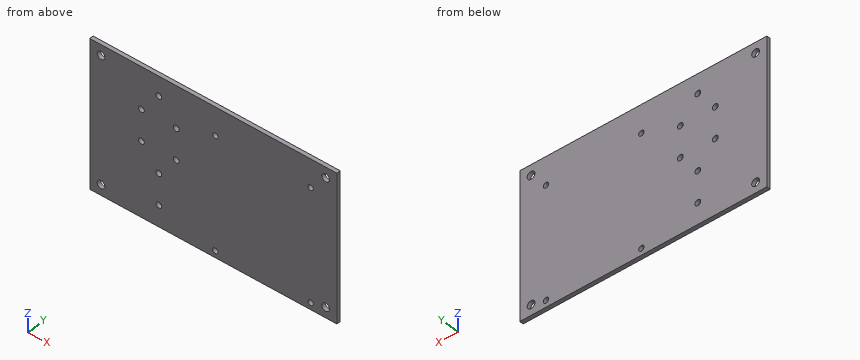
Autodesk Inventor part; units mm, degrees
ref_plane "YZ Plane" through (0, 0, 0) normal (1, 0, 0) x (0, 1, 0)
ref_plane "XZ Plane" through (0, 0, 0) normal (0, 1, 0) x (-1, 0, 0)
ref_plane "XY Plane" through (0, 0, 0) normal (0, 0, 1) x (1, 0, 0)
sketch "Sketch1" plane through (0, 0, 0) normal (0, 1, 0) x (-1, 0, 0)
  line L0 (0, 0) -> (-127, 0)
  line L1 (-127, 0) -> (-127, 76)
  line L2 (-127, 76) -> (0, 76)
  line L3 (0, 76) -> (0, 0)
  dimension "d0" = 76
  dimension "d1" = 127
extrude "Extrusion1" add sketch "Sketch1" along normal blind 2
sketch "Sketch2" plane through (0, 0, 0) normal (0, -1, 0) x (1, 0, 0)
  line L0 (0, 0) -> (127, 0)
  line L1 (127, 0) -> (127, 76)
  line L2 (127, 76) -> (0, 76)
  line L3 (0, 76) -> (0, 0)
  line L4 (0, 5.4) -> (127, 5.4) construction
  line L5 (0, 38) -> (127, 38) construction
  line L6 (63.5, 76) -> (63.5, 0) construction
  line L7 (121.2, 76) -> (121.2, 0) construction
  line L8 (0, 70.6) -> (127, 70.6) construction
  line L9 (5.8, 76) -> (5.8, 0) construction
  circle A0 centre (121.2, 70.6) radius 2
  circle A1 centre (121.2, 5.4) radius 2
  circle A2 centre (5.8, 70.6) radius 2
  circle A3 centre (5.8, 5.4) radius 2
  dimension "d5" = 32.6
  dimension "d6" = 57.7
  dimension "d7" = 4
extrude "Extrusion2" cut sketch "Sketch2" against normal through all contours A0 | A1 | A2 | A3
sketch "Sketch3" plane through (0, 0, 0) normal (0, -1, 0) x (1, 0, 0)
  line L0 (0, 0) -> (127, 0)
  line L1 (0, 76) -> (0, 0)
  line L2 (10, 93) -> (61, 93)
  line L3 (61, 93) -> (61, 0)
  line L4 (61, 0) -> (10, 0)
  line L5 (10, 0) -> (10, 93)
  line L6 (61, 0) -> (117, 0)
  line L7 (117, 0) -> (117, 85)
  line L8 (117, 85) -> (61, 85)
  line L9 (61, 85) -> (61, 0)
  line L10 (35.5, 93) -> (35.5, 0) construction
  circle A0 centre (35.5, 27) radius 1.5
  circle A1 centre (35.5, 82) radius 1.5
  line L11 (89, 85) -> (89, 0) construction
  line L12 (117, 42.5) -> (61, 42.5) construction
  circle A2 centre (113.5, 3.5) radius 1.375
  circle A3 centre (113.5, 61.5) radius 1.375
  circle A4 centre (64.5, 3.5) radius 1.375
  circle A5 centre (64.5, 61.5) radius 1.375
  line L13 (35.5, 82) -> (35.5, 27) construction
  circle A6 centre (44.48, 54.5) radius 1.5
  circle A7 centre (26.52, 54.5) radius 1.5
  circle A8 centre (35.5, 11) radius 1.5
  circle A9 centre (35.5, 66) radius 1.5
  line L14 (35.5, 66) -> (35.5, 11) construction
  circle A10 centre (44.48, 38.5) radius 1.5
  circle A11 centre (26.52, 38.5) radius 1.5
  dimension "d10" = 93
  dimension "d12" = 51
  dimension "d13" = 10
  dimension "d14" = 56
  dimension "d15" = 85
  dimension "d16" = 27
  dimension "d17" = 3
  dimension "d20" = 55
  dimension "d25" = 0
  dimension "d27" = 2.75
  dimension "d31" = 58
  dimension "d34" = 49
  dimension "d39" = 3.5
  dimension "d41" = 3.5
  dimension "d42" = 3
  dimension "d43" = 8.98
  dimension "d44" = 27.5
  dimension "d45" = 3
  dimension "d46" = 55
  dimension "d47" = 3
  dimension "d48" = 27.5
  dimension "d49" = 11
  dimension "d50" = 8.98
  dimension "d51" = 8.98
  dimension "d52" = 3
extrude "Extrusion3" cut sketch "Sketch3" against normal through all contours A0 | A1 | A2 | A3 | A4 | A5 | A6 | A7 | A8 | A9 | A10 | A11
properties part number "base_ps_rpi"
Model file for the job. Use its own axes, mm. Coordinates: 2 decimals unless noted, no trailing zeros. Order: outer loops, then holes, each group sorted by start corner. A loop starts at its lowest first (then second) coordinate and runs counter-clockwise, first axis right, second up. Notation, with made-up numbers: (9, -4) -> (20, -4) arc R12 cw to (20, 0) -> close; hole circle Ø2 at (79, 84.25). An arc over 180 degrees is marked (long way). Return JSON: item names as keys, results as strings. Group by question number.
Item 1: Saw through at B-B on x = 35.5. Write the cut outline in (y, z).
Item 2: Flat gauge pin, fed straight in: P1, Ø2.5, axis at x = 44.48, z = 54.5, coming from the +Y side. Where does the tip first touch, or does it go through?
Item 3: Wall check: line 1 along Z through (x, y) = (26.52, 1.05); line 2 along Z through (x, y) = (64.5, 1.1) (3 decimals); line 3 along X through (y, z) = (1.35, 70.5). Give the ranges that are in metal, low to high. Write a range as [from, to].
Item 4: Saw through at C-C on x = 113.5. Write the cut outline in (y, z) (3 decimals), then the cut area to 3 significant figures.
Item 5: Saw through at A-A on z = 70.6. Write the cut outline in (x, y), then the cut area to 3 significant figures.
Values found:
{
 "1": {"outline": "(0, 0) -> (2, 0) -> (2, 9.5) -> (0, 9.5) -> close; (0, 12.5) -> (2, 12.5) -> (2, 25.5) -> (0, 25.5) -> close; (0, 28.5) -> (2, 28.5) -> (2, 64.5) -> (0, 64.5) -> close; (0, 67.5) -> (2, 67.5) -> (2, 76) -> (0, 76) -> close"},
 "2": {"P1": "passes through"},
 "3": {"line 1": "z = [0, 37], [40, 53], [56, 76]", "line 2": "z = [0, 2.125], [4.875, 60.125], [62.875, 76]", "line 3": "x = [0, 3.8], [7.8, 119.2], [123.2, 127]"},
 "4": {"outline": "(0, 0) -> (2, 0) -> (2, 2.125) -> (0, 2.125) -> close; (0, 4.875) -> (2, 4.875) -> (2, 60.125) -> (0, 60.125) -> close; (0, 62.875) -> (2, 62.875) -> (2, 76) -> (0, 76) -> close", "area": "141 mm2"},
 "5": {"outline": "(0, 0) -> (3.8, 0) -> (3.8, 2) -> (0, 2) -> close; (7.8, 0) -> (119.2, 0) -> (119.2, 2) -> (7.8, 2) -> close; (123.2, 0) -> (127, 0) -> (127, 2) -> (123.2, 2) -> close", "area": "238 mm2"}
}
